```python
from build123d import *

# Parameters (mm, degrees)
SKETCH2_R           = 9.4
BOSS_EXTRUDE1_DEPTH = 24.5
SKETCH3_R           = 3
CUT_EXTRUDE1_DEPTH  = 7.9
SKETCH4_R           = 3.175
CUT_EXTRUDE2_DEPTH  = 16.6


with BuildPart() as part:
    # Sketch2 → Boss-Extrude1 (new body)
    with BuildSketch(Plane(origin=(0, 0, 0), x_dir=(1, 0, 0), z_dir=(0, 1, 0))):
        Circle(SKETCH2_R)
    extrude(amount=BOSS_EXTRUDE1_DEPTH)

    # Sketch3 → Cut-Extrude1 (cut)
    with BuildSketch(Plane(origin=(0, 24.5, 0), x_dir=(1, 0, 0), z_dir=(0, 1, 0))):
        Circle(SKETCH3_R)
    extrude(amount=-CUT_EXTRUDE1_DEPTH, mode=Mode.SUBTRACT)

    # Sketch4 → Cut-Extrude2 (cut)
    with BuildSketch(Plane.XZ):
        Circle(SKETCH4_R)
    extrude(amount=-CUT_EXTRUDE2_DEPTH, mode=Mode.SUBTRACT)


solid = part.part
```
Verification items for the finished model (mm, model axes). Coordinates: 2 decimals unless noted, no trailing zeros. Order: outer loops, then holes, each group sorted by start corner. A loop starts at its lowest first (then second) coordinate and runs counter-clockwise, first axis right, second up. Notation, with made-up numbers: (33.25, 31.5) -> (52.25, 31.5) arc R31 ccw to (52.25, 68.5) -> close; hole circle Ø4 at (61.5, 66.5). An arc over 180 degrees is marked (long way). Answer as CSV lines item,"result". Start each with the question number.
1) Cross-section at D-D, the plane y = 8.75. Record the boundary of the cut face in (x, z) (3 decimals), then the cut area to 3 significant figures.
2) Gauge pin test, flat ends, axial feed: pin 1 Ø3.5 at (x, z) = (0, 0) entering from +Y; pin 2 Ø6 at (y, z) = (6.5, 6.5) entering from -X; pin 3 Ø1 at (x, y) = (1.5, 4.5) entering from -Z. Record the tip position at first contact, or that the pin passes through.
3) Cross-section at C-C, the plane y = 19.5. Record the boundary of the cut face in (x, z), then the cut area to 3 significant figures.
4) Cross-section at A-A, the plane z = 0. Record the boundary of the cut face in (x, y) (3 decimals), then the cut area to 3 significant figures.
5) Material ranges on L1, parallel to X at y = 19, z = 0; L2, parallel to Z at x = 0, y = 9.5 (3 decimals), recorded low to high. Write a range as [from, to].
6) Cross-section at B-B, the plane x = 0. Record the boundary of the cut face in (y, z) (3 decimals).
7) Release check for a two-part mould opening along Z. For faces 1 (the face through (-0.69, 8.18, -3.1)), 2 (the face through (-2.038, 12.078, 9.176)), 3 (the face through (0, 0, 4)) record: released by +Z, released by -Z, zero draft, split by the parting line, or undercut.
Conclusion:
1,outline,"circle Ø18.8 at (0, 0); hole circle Ø6.35 at (0, 0)"
1,area,"246 mm²"
2,pin 1,"passes through"
2,pin 2,"stops at x = -8.72"
2,pin 3,"stops at z = -9.35"
3,outline,"circle Ø18.8 at (0, 0); hole circle Ø6 at (0, 0)"
3,area,"249 mm²"
4,outline,"(-9.4, 0) -> (-3.175, 0) -> (-3.175, 16.6) -> (-3, 16.6) -> (-3, 24.5) -> (-9.4, 24.5) -> close; (3, 16.6) -> (3.175, 16.6) -> (3.175, 0) -> (9.4, 0) -> (9.4, 24.5) -> (3, 24.5) -> close"
4,area,"308 mm²"
5,L1,"x = [-9.4, -3], [3, 9.4]"
5,L2,"z = [-9.4, -3.175], [3.175, 9.4]"
6,outline,"(0, -9.4) -> (24.5, -9.4) -> (24.5, -3) -> (16.6, -3) -> (16.6, -3.175) -> (0, -3.175) -> close; (0, 3.175) -> (16.6, 3.175) -> (16.6, 3) -> (24.5, 3) -> (24.5, 9.4) -> (0, 9.4) -> close"
7,face 1,"undercut"
7,face 2,"split by the parting line"
7,face 3,"zero draft"
